Geometry: see drawing. Coordinates: mm, zero at the bounding-box minimum. A direction names the side the tool comes from. Give positions to 0.01 mm unless a question says otherwise; leave off trailing zeros. Loops run counter-clockwise (first coordinate to the right, second up) from the corner with the lowest first, then second, coordinate; pieces in that order, holes last. Notation, with made-up numbers: (24, -9.5) - (45, -9.5) arc R8 cw to (45, 0.5) - close; hole circle Ø8 at (88.25, -14). An arc over 180 degrees is marked (long way). Use one line per item in the form item = value.
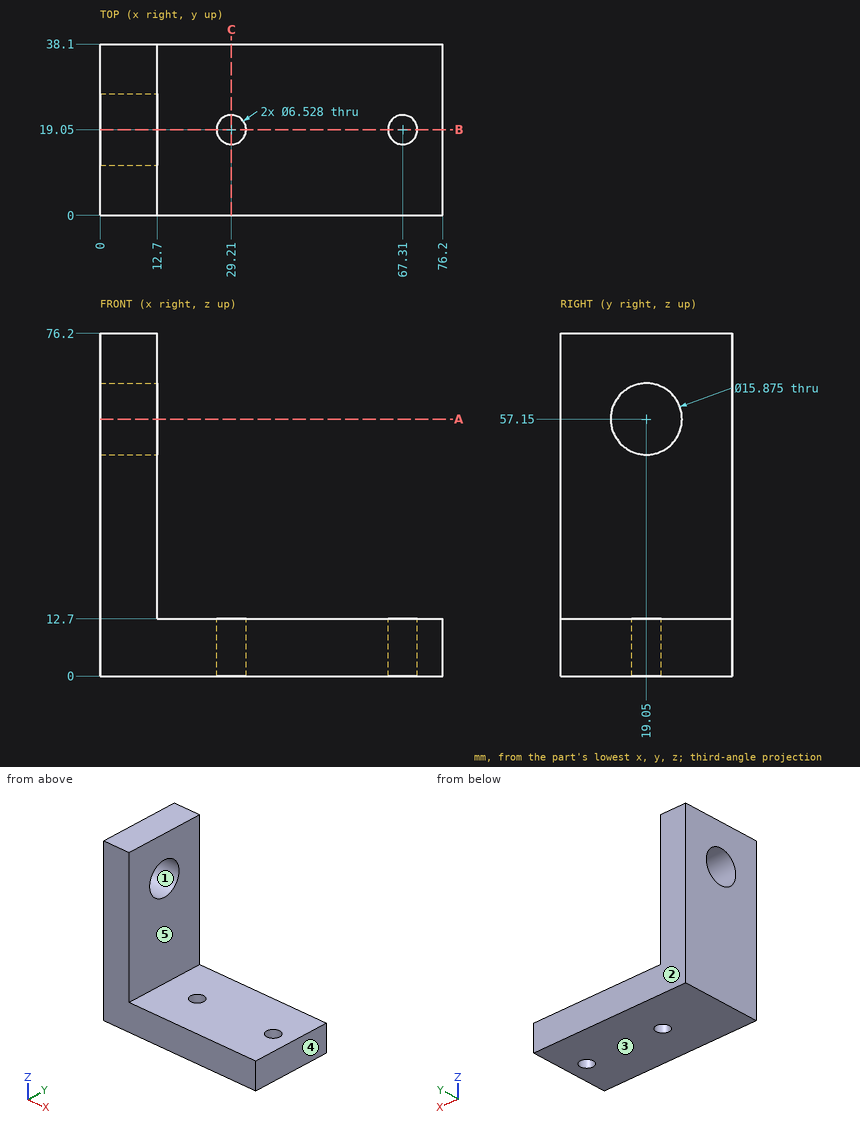
(1) Material intervals for L1, parallel to X at y = 19, z = 9; L2, parallel to Y at x = 29.21, z = 10; L3, parallel to Z at x = 3.5, y = 19, sorted ascending. Write a range as from..to.
Solution:
L1 = 0..25.95, 32.47..64.05, 70.57..76.2
L2 = 0..15.79, 22.31..38.1
L3 = 0..49.21, 65.09..76.2
(2) Cut plane A-A (z = 57.15). Return the cut outline in (x, y).
Solution:
outline = (0, 0) - (12.7, 0) - (12.7, 11.11) - (0, 11.11) - close; (0, 26.99) - (12.7, 26.99) - (12.7, 38.1) - (0, 38.1) - close
(3) Cut plane C-C (x = 29.21). Return the cut outline in (y, z).
Solution:
outline = (0, 0) - (15.79, 0) - (15.79, 12.7) - (0, 12.7) - close; (22.31, 0) - (38.1, 0) - (38.1, 12.7) - (22.31, 12.7) - close
(4) Pull-direction query (Y, two-part tool) for the marked faces 1, 2 and 3; classes: released by +Y, released by -Y, zero draft, split by the parting line, or undercut.
Solution:
face_1 = undercut
face_2 = released by +Y
face_3 = zero draft
(5) Cut plane B-B (y = 19.05). Return the cut outline in (x, z).
Solution:
outline = (0, 0) - (25.95, 0) - (25.95, 12.7) - (12.7, 12.7) - (12.7, 49.21) - (0, 49.21) - close; (0, 65.09) - (12.7, 65.09) - (12.7, 76.2) - (0, 76.2) - close; (32.47, 0) - (64.05, 0) - (64.05, 12.7) - (32.47, 12.7) - close; (70.57, 0) - (76.2, 0) - (76.2, 12.7) - (70.57, 12.7) - close
(6) Pin query (flat end, axial travel): P1, Ø3, axis at y = 25, z = 49.5, coming from the -X side; P2, Ø8.5, axis at x = 29.21, y = 19.05, coming from the +Z side; P3, Ø20.5, axis at y = 19.05, z = 57.15, coming from the +X side. Return the tip coordinate at first contact, or that it passes through.
Solution:
P1 = 0
P2 = 12.7
P3 = 12.7
(7) Access query for the marked faces 4 and 5. Directions: +Z, -Z, +X, -X, +Y, -Y. A direction counts if a zero-diameter tool reaches every point of the face in a straight line with its end or side. Return the directions, or none.
Solution:
face_4 = +Z, -Z, +X, +Y, -Y
face_5 = +Z, +X, +Y, -Y
